```python
from build123d import *

# Parameters (mm, degrees)
ESQUISSE1_R        = 10
BOSS_EXTRU_3_DEPTH = 10


with BuildPart() as part:
    # Esquisse1 → Boss.-Extru.3 (new body)
    with BuildSketch(Plane.XY):
        with BuildLine():
            Line((0, -12.833333333), (-25.552770798, -12.833333333))
            Line((-25.552770798, -12.833333333), (-25.552770798, -10.833333333))
            Line((-25.552770798, -10.833333333), (-12.123210063, -10.833333333))
            ThreePointArc((-12.123210063, -10.833333333), (-10.340577802, -9.740098034), (-10.506782054, -7.655555556))
            ThreePointArc((-10.506782054, -7.655555556), (0, 13), (10.506782054, -7.655555556))
            ThreePointArc((10.506782054, -7.655555556), (10.340577802, -9.740098034), (12.123210063, -10.833333333))
            Line((12.123210063, -10.833333333), (24.447229202, -10.833333333))
            Line((24.447229202, -10.833333333), (24.447229202, -12.833333333))
            Line((24.447229202, -12.833333333), (0, -12.833333333))
        make_face()
        Circle(ESQUISSE1_R, mode=Mode.SUBTRACT)
    extrude(amount=BOSS_EXTRU_3_DEPTH)


solid = part.part
```
Part model, mm, in its own coordinate system. Give positions to 0.01 mm unless a question says otherwise; leave off trailing zeros. Write each loop counter-clockwise with the first axis right and the second up, starting at its lowest first coordinate (ties: lowest second). Pieces come first, ordered by that corner, then holes. Notation, with made-up numbers: M 6,18.5 L 28,18.5 A16 ccw 28,36.5 Z; hole C 31.25,-3.75 d7. An arc over 180 degrees is marked long. Use CSV: the item, a comma, the result in double quotes.
Item 1: Slice it at C-C on z = 4.5. Write the cut outline in (x, y).
Taken from the geometry:
outline,"M -25.55,-12.83 L 24.45,-12.83 L 24.45,-10.83 L 12.12,-10.83 A2 cw 10.51,-7.66 A13 ccw long -10.51,-7.66 A2 cw -12.12,-10.83 L -25.55,-10.83 Z; hole C 0,0 d20"
Item 2: Slice it at B-B on y = 0. Write the cut outline in (x, z).
Taken from the geometry:
outline,"M -13,0 L -10,0 L -10,10 L -13,10 Z; M 10,0 L 13,0 L 13,10 L 10,10 Z"
Item 3: Slice it at A-A on x = 0. Write the cut outline in (y, z).
Taken from the geometry:
outline,"M -12.83,0 L -10,0 L -10,10 L -12.83,10 Z; M 10,0 L 13,0 L 13,10 L 10,10 Z"
Item 4: Slice it at D-D on x = -16. Write the cut outline in (y, z).
Taken from the geometry:
outline,"M -12.83,0 L -10.83,0 L -10.83,10 L -12.83,10 Z"
Item 5: Pin check, flat tips, straight feed: P1, Ø6, axis at y = -5, z = 7.5, coming from the +X side; P2, Ø4, axis at y = -3.5, z = 5.5, coming from the +X side; P3, Ø5, axis at x = -11, z = 1.5, coming from the +Y side. Stop position of each tip, or through.
Taken from the geometry:
P1,"stops at x = 12.85"
P2,"stops at x = 12.91"
P3,"stops at y = 9.84"
Item 6: Drill centre lines: probe 1 along Y at (x, z) = (0, 5.75); probe 2 along X at (y, z) = (-0.25, 1); probe 3 along X at (y, z) = (3.25, 8). Where is each one in solid material? Low to high.
Taken from the geometry:
probe 1,"y = -12.83 to -10, 10 to 13"
probe 2,"x = -13 to -10, 10 to 13"
probe 3,"x = -12.59 to -9.46, 9.46 to 12.59"
Item 7: Pull direction Y, two halves, no side cores. Call faces 1 (the face through (0, -12.833, 5)), 2 (the face through (-0.4, -10.4, 10)), 3 (the face through (0, 13, 5)): +Y half, -Y half, draft (parallel to the pull), parting line (faces both ways), or undercut.
Taken from the geometry:
face 1,"-Y half"
face 2,"draft"
face 3,"undercut"
